The listing builds one solid part. Answer for the finished solid, in the listing's coordinates (mm). A direction names the side the tool comes from. Give positions to 0.01 mm unless a question says otherwise; leave off trailing zeros. Write each loop counter-clockwise with the first axis right and the second up, starting at its lowest first coordinate (ties: lowest second). Pieces come first, ordered by that corner, then holes. Notation, with made-up numbers: (-11, 34) - (6, 34) arc R21 ccw to (6, 42) - close; hole circle Ø9 at (-35.75, 62.5). An arc over 180 degrees is marked (long way). Write each question's results on one line, items separated by ' | '. Start each with the question number.
Q1. For a pull along Z with two mould halves and no side action, classify faces 5 (the face through (898, 497, 25.4)), 6 (the face through (1193, 387, 25.4)), 7 (the face through (584.2, 601, 75)), 8 (the face through (609, 387, 127)) as pulls with the +Z half, pulls with the -Z half, needs draft (parallel to the pull), parting line crosses it, or undercut.
Q2. Find the intervals of material crossed by probe 1 along X at (y, z) = (351, 66); probe 2 along Y at (x, z) = (630, 133); probe 3 along Z at (x, y) = (776, 89), in increasing order.
Q3. Section B-B (z = 97.5) is taken. Determine the outline of the cut face in (x, y).
Q4. For faces 1 (the face through (601, 0, 58)), 2 (the face through (1168.4, 601, 75)), 3 (the face through (1193, 834, 25.4)), 4 (the face through (1193, 834, 127)), determine the directions among +Z, -Z, +X, -X, +Y, -Y from which every point of the face is accessible in a straight line to the end or side of a thin tool.
Q5. Section C-C (y = 1146) is taken. Determine the outline of the cut face in (x, z), plus the area to 3 significant figures.
Q6. A flat-ended cylindrical pin translates along its axis: pin 1 Ø15 at (x, y) = (1201.5, 1073) entering from +Z. Find the tip coordinate at first contact, or state that the pin passes through.
Q7. Section D-D (x = 293) is taken. State how many separate pieces and enclosed holes the cut face has, plus the area to 3 significant figures.
Q8. Section A-A (y = 636) is taken. Determine the outline of the cut face in (x, z).
```python
from build123d import *

# Parameters (mm, degrees)
F1_DEPTH = 25.4
F2_W     = 50.8
F2_H     = 1219.2
F2_W_2   = 25.4
F3_DEPTH = 101.6
F4_W     = 1219.2
F4_H     = 101.6
F5_DEPTH = 25.4
F7_DEPTH = 25.4


with BuildPart() as f1:
    # F0 (on Top) → F1 (new body)
    with BuildSketch(Plane.XY):
        Polygon((0, 101.6), (0, 0), (1219.2, 0), (1219.2, 101.6), (609.6, 101.6), align=None)
    extrude(amount=F1_DEPTH)

    # F2 (on face) → F3 (join)
    with BuildSketch(Plane.XY.offset(25.4)):
        with Locations((25.4, 609.6)):
            Rectangle(F2_W, F2_H)
        with Locations((622.3, 609.6)):
            Rectangle(F2_W_2, F2_H)
        with Locations((596.9, 609.6)):
            Rectangle(F2_W_2, F2_H)
        with Locations((1193.8, 609.6)):
            Rectangle(F2_W, F2_H)
    extrude(amount=F3_DEPTH)

    # F4 (on face) → F5 (join)
    with BuildSketch(Plane.XY.offset(127)):
        with Locations((609.6, 1168.4)):
            Rectangle(F4_W, F4_H)
        with Locations((609.6, 944.88)):
            Rectangle(F4_W, F4_H)
        with Locations((609.6, 721.36)):
            Rectangle(F4_W, F4_H)
        with Locations((609.6, 497.84)):
            Rectangle(F4_W, F4_H)
        with Locations((609.6, 274.32)):
            Rectangle(F4_W, F4_H)
        with Locations((609.6, 50.8)):
            Rectangle(F4_W, F4_H)
    extrude(amount=F5_DEPTH)

    # F6 (on face) → F7 (join)
    with BuildSketch(Plane(origin=(0, 0, 25.4), x_dir=(1, 0, 0), z_dir=(0, 0, -1))):
        Polygon((0, -325.12), (609.6, -325.12), (1219.2, -325.12), (1219.2, -223.52), (609.6, -223.52), (0, -223.52), align=None)
        Polygon((0, -447.04), (0, -548.64), (609.6, -548.64), (1219.2, -548.64), (1219.2, -447.04), (609.6, -447.04), align=None)
        Polygon((0, -670.56), (0, -772.16), (609.6, -772.16), (1219.2, -772.16), (1219.2, -670.56), (609.6, -670.56), align=None)
        Polygon((0, -894.08), (0, -995.68), (609.6, -995.68), (1219.2, -995.68), (1219.2, -894.08), (609.6, -894.08), align=None)
        Polygon((0, -1219.2), (1219.2, -1219.2), (1219.2, -1117.6), (609.6, -1117.6), (0, -1117.6), align=None)
    extrude(amount=F7_DEPTH)


solid = f1.part
```
Answers below:
1) face 5: undercut | face 6: pulls with the -Z half | face 7: undercut | face 8: pulls with the +Z half
2) probe 1: x = 0 to 50.8, 584.2 to 635, 1168.4 to 1219.2 | probe 2: y = 0 to 101.6, 223.52 to 325.12, 447.04 to 548.64, 670.56 to 772.16, 894.08 to 995.68, 1117.6 to 1219.2 | probe 3: z = 0 to 25.4, 127 to 152.4
3) outline: (0, 0) - (50.8, 0) - (50.8, 1219.2) - (0, 1219.2) - close; (584.2, 0) - (635, 0) - (635, 1219.2) - (584.2, 1219.2) - close; (1168.4, 0) - (1219.2, 0) - (1219.2, 1219.2) - (1168.4, 1219.2) - close
4) face 1: +Z, -Z, +X, -X, -Y | face 2: +Y, -Y | face 3: -Z, +X, -X | face 4: +Z, +X, -X
5) outline: (0, 0) - (1219.2, 0) - (1219.2, 152.4) - (0, 152.4) - close; hole (50.8, 25.4) - (584.2, 25.4) - (584.2, 127) - (50.8, 127) - close; hole (635, 25.4) - (1168.4, 25.4) - (1168.4, 127) - (635, 127) - close | area: 77,400 mm2
6) pin 1: stops at z = 127
7) separate pieces: 12 | enclosed holes: 0 | area: 31,000 mm2
8) outline: (0, 25.4) - (50.8, 25.4) - (50.8, 127) - (0, 127) - close; (584.2, 25.4) - (635, 25.4) - (635, 127) - (584.2, 127) - close; (1168.4, 25.4) - (1219.2, 25.4) - (1219.2, 127) - (1168.4, 127) - close
